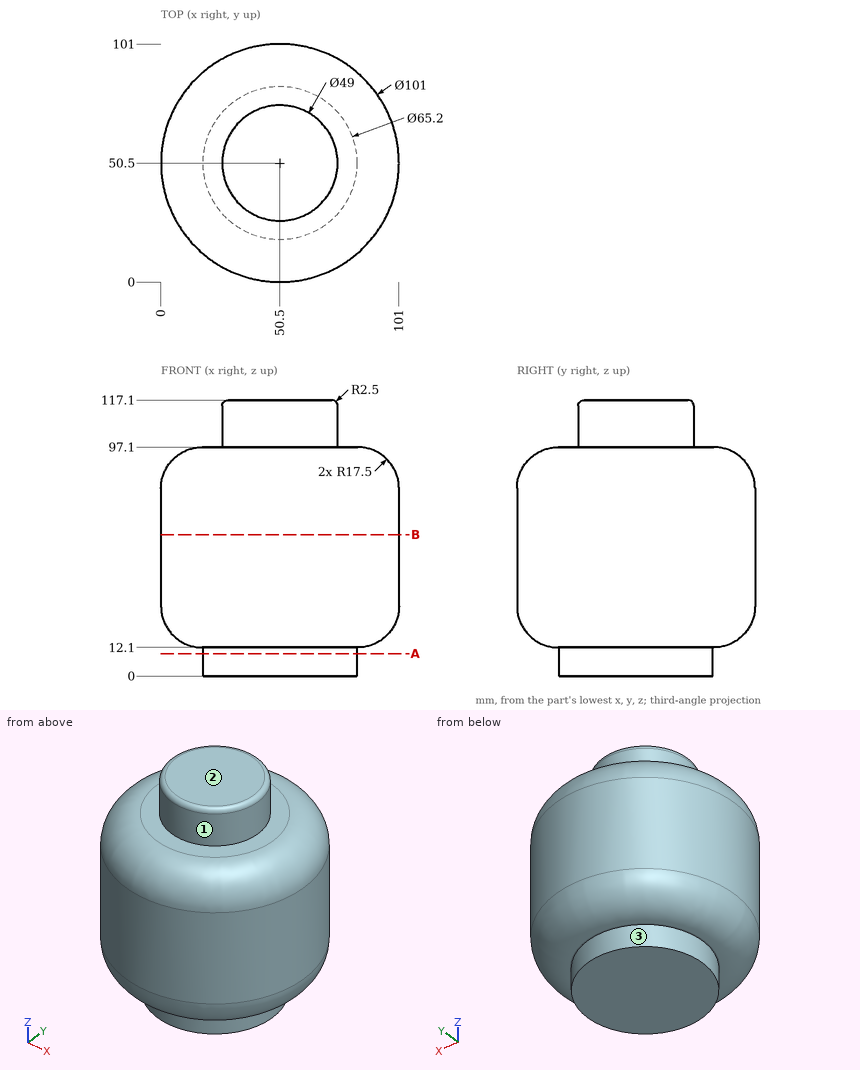
Could you check a few things on this drawing? It's one solid part, dimensions in mm from its lowest x, y, z. A direction names the side the tool comes from. Give positions to 0.01 mm unless a question says otherwise; leave off trailing zeros. Order: outer loops, then holes, each group sorted by start corner. A loop starts at its lowest first (then second) coordinate and runs counter-clockwise, first axis right, second up. Notation, with made-up numbers: (53.25, 70) - (96.25, 70) arc R24 ccw to (96.25, 87) - close; hole circle Ø11 at (-24.75, 18.25). An arc over 180 degrees is marked (long way). Return JSON: item names as keys, results as strings. Group by question number.
Q1. Please list where these lines run through material, in increasing order: line 1 along Z through (x, y) = (66, 73.5); line 2 along X through (y, z) = (49.5, 76.5); line 3 along Z through (x, y) = (15, 66). Write a range as [from, to].
Q2. Which directions (+Z, -Z, +X, -X, +Y, -Y) give clear straight access to the entire face, cutting with the end or side of a thin tool? Please do the marked faces 1, 2 and 3.
Q3. Suppose I cut it at B-B, the plane z = 60. Please give me the cut outline in (x, y).
Q4. Suppose I cut it at A-A, the plane z = 9.5. Please give me the cut outline in (x, y).
Q5. Will these pins go through, and if not, where does the flat tip stop? pin 1 Ø4 at (y, z) = (34.5, 61.5) entering from -X; pin 2 Ø12 at (x, z) = (10.5, 45) entering from -Y; pin 3 Ø3 at (x, y) = (65.5, 13) entering from -Z.
Resolved:
{
 "1": {"line 1": "z = [0, 97.1]", "line 2": "x = [0.01, 100.99]", "line 3": "z = [13.07, 96.13]"},
 "2": {"face 1": "+Z", "face 2": "+Z, +X, -X, +Y, -Y", "face 3": "-Z"},
 "3": {"outline": "circle Ø101 at (50.5, 50.5)"},
 "4": {"outline": "circle Ø65.2 at (50.5, 50.5)"},
 "5": {"pin 1": "stops at x = 1.98", "pin 2": "stops at y = 13.16", "pin 3": "stops at z = 13.12"}
}
